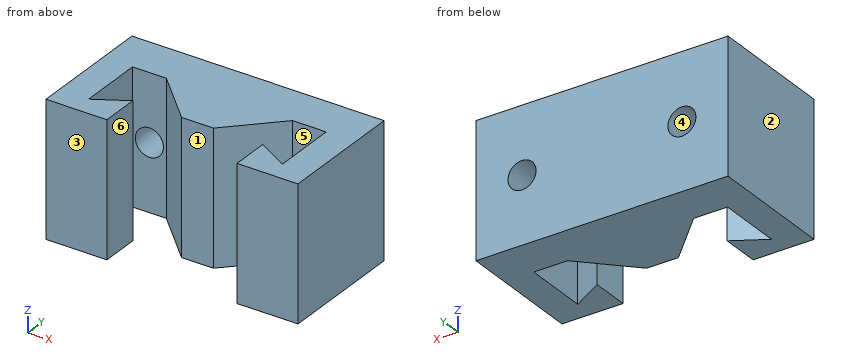
```python
from build123d import *

# Parameters (mm, degrees)
BOSS_EXTRUDE1_DEPTH     = 10
SKETCH2_R               = 2.1
CUT_EXTRUDE1_DEPTH      = 6.35
SKETCH3_W               = 9.725
SKETCH3_H               = 19.05
CUT_EXTRUDE2_DEPTH      = 11
CUT_EXTRUDE2_DEPTH_BACK = 11


with BuildPart() as part:
    # Sketch1 → Boss-Extrude1 (new body, symmetric)
    with BuildSketch(Plane.XY):
        Polygon((9.725, 0), (19.05, 0), (19.05, 19.05), (-19.05, 19.05), (-19.05, 0), (-9.725, 0), (-9.725, 5.724630657), (-14.4875, 2.975), (-14.4875, 12.7), (-9.425, 12.7), (-2.38125, 5.65625), (2.38125, 5.65625), (9.425, 12.7), (14.4875, 12.7), (14.4875, 2.975), (9.725, 5.724630657), align=None)
    extrude(amount=BOSS_EXTRUDE1_DEPTH, both=True)

    # Sketch2 → Cut-Extrude1 (cut)
    with BuildSketch(Plane(origin=(0, 19.05, 0), x_dir=(1, 0, 0), z_dir=(0, 1, 0))):
        with Locations((-11.95625, 0)):
            Circle(SKETCH2_R)
        with Locations((11.95625, 0)):
            Circle(SKETCH2_R)
    extrude(amount=-CUT_EXTRUDE1_DEPTH, mode=Mode.SUBTRACT)

    # Sketch3 → Cut-Extrude2 (cut, two sides)
    with BuildSketch(Plane.XY) as cut_extrude2_sk:
        with Locations((-23.7125, 9.525)):
            Rectangle(SKETCH3_W, SKETCH3_H)
        with Locations((23.7125, 9.525)):
            Rectangle(SKETCH3_W, SKETCH3_H)
    extrude(amount=CUT_EXTRUDE2_DEPTH, mode=Mode.SUBTRACT)
    extrude(cut_extrude2_sk.sketch, amount=-CUT_EXTRUDE2_DEPTH_BACK, mode=Mode.SUBTRACT)


solid = part.part
```
Design review of the part built by this model. Coordinates are the model's own, in mm. Face numbers are marked on the shaded views. A direction names the side the tool comes from. Coordinates: 2 decimals unless noted, no trailing zeros. Order: outer loops, then holes, each group sorted by start corner. A loop starts at its lowest first (then second) coordinate and runs counter-clockwise, first axis right, second up. Notation, with made-up numbers: M 87,76 L 111,76 A19 ccw 111,102 Z; hole C 45.5,-33.5 d7. An arc over 180 degrees is marked long. Answer as a JSON object with one key per item and string values. Group by question number.
1) Add section A-A, the plane z = 0. Count the separate pieces of the cut face and the enclosed holes in it, then the cut area to 3 significant figures.
2) Mouldability with a two-part tool opening along X and no side actions: class the marked faces 1, 2 and 3 as pulls with the +X half, pulls with the -X half, needs draft (parallel to the pull), parting line crosses it, or undercut.
3) Tool access review of the marked faces 4, 5 and 6: name each direction out of +Z, -Z, +X, -X, +Y, -Y from which nothing blocks a thin tool from reaching the whole face with its end or side.
4) Add section B-B, the plane y = 18. Write out the cut boundary in (x, z).
5) For pin 1 (4 mm diameter, centred on x = 8, y = 10.5, fed in from -Z); pin 2 (1 mm diameter, centred on x = 0, y = 3.5, fed in from +Z); pin 3 (5 mm diameter, centred on x = 0, z = 0.5, fed in from -Y), all flat-tipped, find the tip position at first contact; note any pin that passes through.
6) Wall thickness on L1, parallel to X at y = 15.25, z = 0; L2, parallel to X at y = 1.5, z = -9 (3 decimals); L3, parallel to X at y = 14, z = -1: over which ranges is each line inside the solid? List them lowest first.
Computed values:
{
 "1": {"separate pieces": "3", "enclosed holes": "0", "area": "421 mm^2"},
 "2": {"face 1": "undercut", "face 2": "pulls with the -X half", "face 3": "needs draft"},
 "3": {"face 4": "+Y", "face 5": "+Z, -Z", "face 6": "+Z, -Z, -Y"},
 "4": {"outline": "M -18.85,-10 L 18.85,-10 L 18.85,10 L -18.85,10 Z; hole C -11.96,0 d4.2; hole C 11.96,0 d4.2"},
 "5": {"pin 1": "stops at z = -10", "pin 2": "passes through", "pin 3": "stops at y = 5.66"},
 "6": {"L1": "x = -18.85 to -14.06, -9.86 to 9.86, 14.06 to 18.85", "L2": "x = -18.85 to -9.725, 9.725 to 18.85", "L3": "x = -18.85 to -13.8, -10.11 to 10.11, 13.8 to 18.85"}
}
